Geometry check sheet. Reference: the model listing, model coordinates, mm. A direction names the side the tool comes from. Give positions to 0.01 mm unless a question says otherwise; leave off trailing zeros. Write item = value, one per line. Start each with the question number.
(1) Draft check along Y on faces 1 (the flat face through (2, 0, -3)), 2 (the flat face through (-7.75, 256, 0)), 3 (the flat face through (-2.35, 71.8, 2.2)), 4 (the flat face through (0, 520, 0)). Enter one of: pulls with the +Y half, pulls with the -Y half, needs draft (parallel to the pull), parting line crosses it, or undercut.
(2) Thickness scan on L1, parallel to Y at x = 4.5, z = 0; L2, parallel to Y at x = -5.1, z = 0; L3, parallel to Z at x = 1, y = 232.5. Record the ranges inside material, lowest first.
(3) Depth check by flat-ended pin: pin 1 Ø3 at (y, z) = (71.5, -1) entering from -X; pin 2 Ø3.5 at (y, z) = (232, 0) entering from +X. Enter the tip coordinate at first touch or a pass-through.
(4) Access from +Z, -Z, +X, -X, +Y, -Y to the whole of each face (thin tool, end or side, straight path). Record for faces 5 (the cylindrical face through (-5.09, 69.12, -1.08)), 6 (the flat face through (0, 254, -12.5)).
```python
from build123d import *

# Parameters (mm, degrees)
SKETCH1_W                                           = 15.5
SKETCH1_H                                           = 25
BOSS_EXTRUDE1_DEPTH                                 = 520
FILLET1_R                                           = 5
F_5_0MM_DOWEL_HOLE1_D                               = 6.6
F_5_0MM_DOWEL_HOLE1_DEPTH                           = 12
F_5_0MM_DOWEL_HOLE1_TIP                             = 1.982840043
CBORE_FOR_M5_HEX_SOCKET_HEAD_CAP_SCREW2_D           = 5.5
CBORE_FOR_M5_HEX_SOCKET_HEAD_CAP_SCREW2_CBORE_D     = 10
CBORE_FOR_M5_HEX_SOCKET_HEAD_CAP_SCREW2_CBORE_DEPTH = 5.4


with BuildPart() as part:
    # Sketch1 → Boss-Extrude1 (new body)
    with BuildSketch(Plane(origin=(0, 0, 0), x_dir=(1, 0, 0), z_dir=(0, 1, 0))):
        Rectangle(SKETCH1_W, SKETCH1_H)
    extrude(amount=BOSS_EXTRUDE1_DEPTH)

    # Fillet1
    fillet1_edges = [part.edges().sort_by_distance(p)[0] for p in [
        (0, 520, -12.5),
        (0, 520, 12.5),
    ]]
    fillet(fillet1_edges, radius=FILLET1_R)

    # Ø5.0mm Dowel Hole1
    with Locations(Plane(origin=(0, 0, 0), x_dir=(-1, 0, 0), z_dir=(0, -1, 0))):
        with Locations((0, 0)):
            Hole(F_5_0MM_DOWEL_HOLE1_D / 2, depth=F_5_0MM_DOWEL_HOLE1_DEPTH)
            with Locations((0, 0, -(F_5_0MM_DOWEL_HOLE1_DEPTH + F_5_0MM_DOWEL_HOLE1_TIP / 2))):  # 118° drill point
                Cone(0, F_5_0MM_DOWEL_HOLE1_D / 2, F_5_0MM_DOWEL_HOLE1_TIP, mode=Mode.SUBTRACT)

    # CBORE for M5 Hex Socket Head Cap Screw2 (through all)
    with Locations(Plane.ZY.offset(7.75)):
        with Locations((0, 74), (0, 232)):
            CounterBoreHole(CBORE_FOR_M5_HEX_SOCKET_HEAD_CAP_SCREW2_D / 2, CBORE_FOR_M5_HEX_SOCKET_HEAD_CAP_SCREW2_CBORE_D / 2, CBORE_FOR_M5_HEX_SOCKET_HEAD_CAP_SCREW2_CBORE_DEPTH)


solid = part.part
```
Model answer:
q1.face_1 = pulls with the -Y half
q1.face_2 = needs draft
q1.face_3 = undercut
q1.face_4 = pulls with the +Y half
q2.L1 = 0 to 71.25, 76.75 to 229.25, 234.75 to 520
q2.L2 = 0 to 69, 79 to 227, 237 to 520
q2.L3 = -12.5 to -2.7, 2.7 to 12.5
q3.pin_1 = -2.35
q3.pin_2 = through
q4.face_5 = -X
q4.face_6 = -Z, +X, -X, +Y, -Y
